Geometry: final body of the model. Coordinates: model frame, mm. A direction names the side the tool comes from. Give positions to 0.01 mm unless a question says otherwise; leave off trailing zeros. Loops run counter-clockwise (first coordinate to the right, second up) from the corner with the lowest first, then second, coordinate; pieces in that order, holes last.
1. First-contact query: P1, Ø1.6, axis at y = -3, z = 10.5, coming from the +X side; P2, Ø0.8, axis at x = -48, y = -1, coming from the -Z side; P3, Ø2, axis at x = -58, y = -3, coming from the +Z side; P4, Ø1.3, axis at x = -63.49, y = -3.5, coming from the -Z side. Flat tips, straight axial feed; report the tip coordinate or a pass-through.
2. Section B-B, the plane x = -57.5. Output: boundary loops of the cut face in (y, z), then the cut area to 3 significant figures.
3. Material intervals for line 1 along X through (y, z) = (-3.5, -2.5); line 2 along Y through (x, z) = (-49, 7.5); line 3 along Z through (x, y) = (-43.5, -5), sorted ascending.
4. Access query for faces 5 (the face through (-60, -4, -1.5)), 6 (the face through (-33.31, -3.47, -2.77)), 7 (the face through (-43.75, -3, 7)), 8 (the face through (-32.01, -3.46, -2.77)), 9 (the face through (-49, -1, 8.5)). Directions: +Z, -Z, +X, -X, +Y, -Y. A direction counts if a zero-diameter tool reaches every point of the face in a straight line with its end or side. Return the directions, or none.
5. Section A-A, the plane y = -3.5. Output: boundary loops of the cut face in (x, z).
6. Section C-C, the plane z = 4. Output: boundary loops of the cut face in (x, y).
7. Draft query along Y for faces 1 (the face through (-63, -3, -3)), 2 (the face through (-65.49, -3.54, -2.77)), 3 (the face through (-44.32, -2.79, 17.9)), 4 (the face through (-49, -1.5, 1)). Return one class per face: +Y half, -Y half, draft (parallel to the pull), parting line (faces both ways), or undercut.
8. Section D-D, the plane x = -45. Output: boundary loops of the cut face in (y, z).
Autodesk Inventor part; units mm, degrees
ref_plane "Work Plane1" through (-43.75, 3, -4) normal (0, 0, 1) x (-1, 0, 0)
ref_plane "YZ Plane" through (0, 0, 0) normal (1, 0, 0) x (0, 1, 0)
ref_plane "XZ Plane" through (0, 0, 0) normal (0, 1, 0) x (-1, 0, 0)
ref_plane "Work Plane1" through (-43.75, 3, -4) normal (0, 0, 1) x (-1, 0, 0)
sketch "Sketch1" plane through (-43.75, 3, -4) normal (0, 0, 1) x (-1, 0, 0)
  circle A0 centre (-9.7413, 6.5) radius 0.7
  circle A1 centre (19.7413, 6.5) radius 0.7
  circle A2 centre (-9.7413, 6.5) radius 2
  circle A3 centre (19.7413, 6.5) radius 2
  line L0 (-9.7413, 8.5) -> (19.7413, 8.5)
  line L1 (-9.7413, 4.5) -> (19.7413, 4.5)
  point P0 (-43.75, 3)
  dimension "d0" = 4
  dimension "d1" = 4
extrude "Extrusion1" add sketch "Sketch1" along normal blind 2.5
sketch "Sketch2" plane through (-43.75, 3, -1.5) normal (0, 0, 1) x (1, 0, 0)
  line L0 (9.7413, -4.5) -> (-19.7413, -4.5)
  line L1 (-19.7413, -8.5) -> (9.7413, -8.5)
  line L2 (-10, -4.5) -> (0, -4.5)
  line L3 (0, -4.5) -> (0, -8.5)
  line L4 (0, -8.5) -> (-10, -8.5)
  line L5 (-10, -8.5) -> (-10, -4.5)
  circle A0 centre (-5, -6.5) radius 1.25
  point P0 (43.75, -3)
  dimension "d4" = 10
  dimension "d6" = 5
extrude "Extrusion2" add sketch "Sketch2" along normal blind 20 contours L3 L1 L5 L0 | A0
sketch "Sketch3" plane through (-63.4913, -1.5, -4) normal (0, 1, 0) x (1, 0, 0)
  line L0 (19.7413, -2.5) -> (19.7413, -22.5)
  line L1 (9.7413, -22.5) -> (19.7413, -22.5)
  line L2 (19.7413, -22.5) -> (19.7413, -12.5)
  line L3 (19.7413, -12.5) -> (9.7413, -12.5)
  line L4 (9.7413, -12.5) -> (9.7413, -22.5)
  point P0 (63.4913, -4)
extrude "Extrusion3" add sketch "Sketch3" along normal blind 1.5
fillet "Fillet1" radius 2 2 edges at (-53.75, -2.75, 18.5) (-43.75, -2.75, 18.5)
properties part number "HornBase"
Answers below:
1. P1: stops at x = -43.75
1. P2: stops at z = 8.5
1. P3: stops at z = -1.5
1. P4: passes through
2. outline: (-5.5, -4) - (-1.5, -4) - (-1.5, -1.5) - (-5.5, -1.5) - close
2. area: 10.0 mm2
3. line 1: x = -65.49 to -64.19, -62.79 to -34.71, -33.31 to -32.01
3. line 2: y = -5.5 to -1.5
3. line 3: z = -4 to -1.5
4. face 5: +Z, -X, +Y, -Y
4. face 6: +Z, -Z
4. face 7: +Z, +X, +Y, -Y
4. face 8: +Z, -Z, +X
4. face 9: -Z, +X, -X, +Y
5. outline: (-65.49, -4) - (-64.19, -4) - (-64.19, -1.5) - (-65.49, -1.5) - close; (-62.79, -4) - (-34.71, -4) - (-34.71, -1.5) - (-43.75, -1.5) - (-43.75, 16.5) arc R2 ccw to (-45.75, 18.5) - (-51.75, 18.5) arc R2 ccw to (-53.75, 16.5) - (-53.75, -1.5) - (-62.79, -1.5) - close; (-33.31, -4) - (-32.01, -4) - (-32.01, -1.5) - (-33.31, -1.5) - close
6. outline: (-53.75, -5.5) - (-43.75, -5.5) - (-43.75, -1.5) - (-53.75, -1.5) - close
7. face 1: undercut
7. face 2: parting line
7. face 3: draft
7. face 4: +Y half
8. outline: (-5.5, -4) - (-1.5, -4) - (-1.5, 8.5) - (0, 8.5) - (0, 18.35) - (-5.5, 18.35) - close
